Check sheet for the modelled part. Datum: model origin and axes. Units: mm. Face numbers are marked on the shaded views. A direction names the side the tool comes from. Coordinates: 2 decimals unless noted, no trailing zeros. Loops run counter-clockwise (first coordinate to the right, second up) from the corner with the lowest first, then second, coordinate; pieces in that order, holes last. Notation, with made-up numbers: M 86,-40 L 144,-40 A19 ccw 144,-25 Z; hole C 34.25,55.25 d10. An arc over 180 degrees is marked long. Return JSON: item names as keys, results as strings.
from build123d import *

# Parameters (mm, degrees)
F0_R     = 9.1559693167
F1_DEPTH = 50
F2_R     = 20
F3_R     = 5
F4_R     = 5
F5_R     = 5


with BuildPart() as f1:
    # F0 (on Front) → F1 (new body)
    with BuildSketch(Plane.XZ):
        Polygon((-26.2572392821, 58.8964447379), (-30.6334458292, 23.8867942244), (-55.4319471121, -8.5700713098), (-24.0691360086, -37.0154157281), (-18.469100818, -12.2761549428), (-9.3532412677, -28.9885639891), (16.0460937768, -15.1343811303), (29.9040805548, -33.7332598865), (53.9732128382, 25.7102139294), (26.6219247133, 20.239956677), (17.8695097566, 65.4607564211), align=None)
        with Locations((-9.1187059879, 34.7417481244)):
            Circle(F0_R, mode=Mode.SUBTRACT)
    extrude(amount=F1_DEPTH)

    # F2
    f2_edges = [f1.edges().sort_by_distance(p)[0] for p in [
        (-55.431947, -25, -8.570071),
    ]]
    fillet(f2_edges, radius=F2_R)

    # F3
    f3_edges = [f1.edges().sort_by_distance(p)[0] for p in [
        (-26.257239, -25, 58.896445),
    ]]
    fillet(f3_edges, radius=F3_R)

    # F4
    f4_edges = [f1.edges().sort_by_distance(p)[0] for p in [
        (-37.452482, -50, 14.961878),
        (-48.296803, -50, -7.920016),
        (-2.31645, -50, 62.457885),
        (22.245717, -50, 42.850357),
        (40.297569, -50, 22.975085),
        (-28.68077, -50, 39.508202),
        (-25.343225, -50, 58.003503),
        (-32.942365, -50, -28.967603),
        (-21.269118, -50, -24.645785),
        (41.938647, -50, -4.011523),
        (-13.911171, -50, -20.632359),
        (22.975087, -50, -24.433821),
        (3.346426, -50, -22.061473),
        (-18.274675, -50, 34.741748),
    ]]
    fillet(f4_edges, radius=F4_R)

    # F5
    f5_edges = [f1.edges().sort_by_distance(p)[0] for p in [
        (22.245717, 0, 42.850357),
        (-2.31645, 0, 62.457885),
        (-25.343225, 0, 58.003503),
        (-28.68077, 0, 39.508202),
        (-37.452482, 0, 14.961878),
        (-48.296803, 0, -7.920016),
        (-32.942365, 0, -28.967603),
        (40.297569, 0, 22.975085),
        (-21.269118, 0, -24.645785),
        (41.938647, 0, -4.011523),
        (-13.911171, 0, -20.632359),
        (22.975087, 0, -24.433821),
        (3.346426, 0, -22.061473),
        (-18.274675, 0, 34.741748),
    ]]
    fillet(f5_edges, radius=F5_R)


solid = f1.part
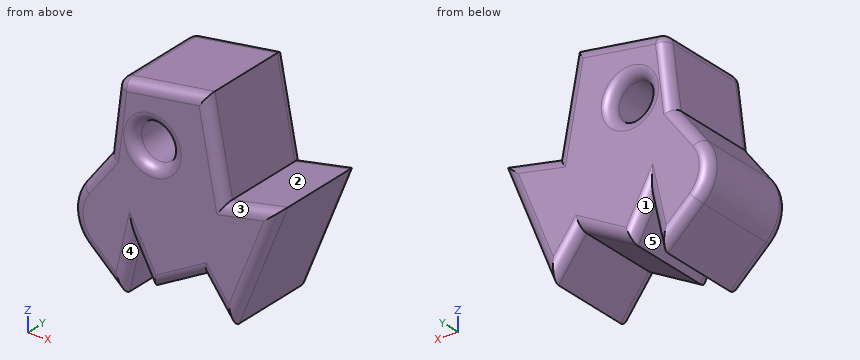
1) Set-up check for the marked faces 1, 2, 3, 4 and 5: record each of +Z, -Z, +X, -X, +Y, -Y from which the full face is reachable in a straight line by a thin tool's end or side.
Answers:
{"face 1": "-Z, +Y", "face 2": "+Z, +Y, -Y", "face 3": "+Z, -Y", "face 4": "-Z, -Y", "face 5": "-Z, +Y, -Y"}
2) Scan lines: line 1 along X through (y, z) = (-11.5, -23); line 2 along X through (y, z) = (-4, -21); line 3 along Y through (x, z) = (-22, -7). Record each from-to range of solid material in increasing order. Write a range as [from, to].
Answers:
{"line 1": "[-39.52, -20.9], [-12.62, 1.63], [21.91, 34.25]", "line 2": "[-41.58, -20.55], [-13.6, 5.08], [20.54, 34.95]", "line 3": "[-49.98, -0.02]"}
3) Section check A-A on y = -8. Record the cut outline in (x, z), then the cut area to 3 significant figures.
Answers:
{"outline": "M -44.27,6.04 A20 ccw -41.82,-20.92 L -24.07,-37.02 L -18.47,-12.28 L -9.35,-28.99 L 16.05,-15.13 L 29.9,-33.73 L 53.97,25.71 L 26.62,20.24 L 17.87,65.46 L -22.5,59.46 A5 ccw -26.73,55.13 L -30.63,23.89 Z; hole C -9.12,34.74 d18.31", "area": "5,820 mm²"}
4) Go/stop test with flat-tipped pins: pin 1 Ø10 at (x, y) = (11.5, -16.5) entering from -Z; pin 2 Ø14.5 at (x, z) = (-9.12, 34.74) entering from +Y; pin 3 Ø10 at (x, y) = (-30.5, -34.5) entering from -Z; pin 4 Ø3 at (x, y) = (-14, -16.5) entering from +Z. Record where each tip stops, or that it passes through.
Answers:
{"pin 1": "z = -20.34", "pin 2": "through", "pin 3": "z = -35.72", "pin 4": "z = 60.94"}
